from build123d import *

# Parameters (mm, degrees)
F0_W      = 80
F0_H      = 80
F1_DEPTH  = 20
F2_W      = 75
F2_H      = 75
F3_DEPTH  = 15
F4_R      = 2.5
F4_R_2    = 1.5
F5_DEPTH  = 12
F6_W      = 7.5
F6_H      = 7.5
F7_DEPTH  = 7.5
F8_R      = 2.5
F9_DEPTH  = 15
F10_SIZE2 = 1.4004150764
F10_SIZE  = 2


with BuildPart() as f1:
    # F0 (on Top) → F1 (new body)
    with BuildSketch(Plane.XY):
        Rectangle(F0_W, F0_H)
    extrude(amount=F1_DEPTH)

    # F2 (on face) → F3 (cut)
    with BuildSketch(Plane.XY.offset(20)):
        Rectangle(F2_W, F2_H)
    extrude(amount=-F3_DEPTH, mode=Mode.SUBTRACT)

    # F4 (on face) → F5 (join)
    with BuildSketch(Plane.XY.offset(5)):
        with Locations((-11, 26.5)):
            Circle(F4_R)
        with Locations((-11, 26.5)):
            Circle(F4_R_2, mode=Mode.SUBTRACT)
        with Locations((11, 26.5)):
            Circle(F4_R)
        with Locations((11, 26.5)):
            Circle(F4_R_2, mode=Mode.SUBTRACT)
        with Locations((-11, -26.5)):
            Circle(F4_R)
        with Locations((-11, -26.5)):
            Circle(F4_R_2, mode=Mode.SUBTRACT)
        with Locations((11, -26.5)):
            Circle(F4_R)
        with Locations((11, -26.5)):
            Circle(F4_R_2, mode=Mode.SUBTRACT)
        with Locations((-32.5, 18)):
            Circle(F4_R)
        with Locations((-32.5, 18)):
            Circle(F4_R_2, mode=Mode.SUBTRACT)
        with Locations((-32.5, 0)):
            Circle(F4_R)
        with Locations((-32.5, 0)):
            Circle(F4_R_2, mode=Mode.SUBTRACT)
        with Locations((-32.5, -18)):
            Circle(F4_R)
        with Locations((-32.5, -18)):
            Circle(F4_R_2, mode=Mode.SUBTRACT)
        with Locations((32.5, 0)):
            Circle(F4_R)
        with Locations((32.5, 0)):
            Circle(F4_R_2, mode=Mode.SUBTRACT)
        with Locations((32.5, -18)):
            Circle(F4_R)
        with Locations((32.5, -18)):
            Circle(F4_R_2, mode=Mode.SUBTRACT)
        with Locations((32.5, 18)):
            Circle(F4_R)
        with Locations((32.5, 18)):
            Circle(F4_R_2, mode=Mode.SUBTRACT)
    extrude(amount=F5_DEPTH)

    # F6 (on face) → F7 (join)
    with BuildSketch(Plane(origin=(-40, 0, 0), x_dir=(0, -1, 0), z_dir=(-1, 0, 0))):
        with Locations((35, 15)):
            Rectangle(F6_W, F6_H)
        with Locations((-5, 15)):
            Rectangle(F6_W, F6_H)
    extrude(amount=F7_DEPTH)

    # F8 (on face) → F9 (join)
    with BuildSketch(Plane(origin=(0, -31.25, 0), x_dir=(-1, 0, 0), z_dir=(0, 1, 0))):
        with Locations((43.75, 15)):
            Circle(F8_R)
    extrude(amount=F9_DEPTH)

    # F10
    f10_edges = [f1.edges().sort_by_distance(p)[0] for p in [
        (-41.25, -16.25, 15),
    ]]
    f10_side = f1.faces().sort_by_distance((-43.75, -16.25, 15))[0]
    chamfer(f10_edges, length=F10_SIZE, length2=F10_SIZE2, reference=f10_side)


solid = f1.part
Here's how the part is built. I have some questions about the finished solid (model axes, mm). A direction names the side the tool comes from. Coordinates: 2 decimals unless noted, no trailing zeros. Order: outer loops, then holes, each group sorted by start corner. A loop starts at its lowest first (then second) coordinate and runs counter-clockwise, first axis right, second up. Notation, with made-up numbers: (-2.75, -34.75) - (26.25, -34.75) arc R23 ccw to (26.25, -23.75) - close; hole circle Ø1 at (32.25, 62). An arc over 180 degrees is marked (long way). Use CSV: the item, a comma, the result in double quotes. Start each with the question number.
1. Suppose I cut it at A-A on y = -22.5. List the corners of the cut face in (x, z) for me, then the cut area to 3 significant figures.
2. For faces 1 (the face through (-35, -18, 11)), 2 (the face through (40, -1, 10)), 3 (the face through (-44, 5, 18.75)), 4 (the face through (-46.06, -24.55, 14.04)), which set-ups out of +Z, -Z, +X, -X, +Y, -Y let a thin tool reach every point of the face, with its end or its side?
3. Please list where these lines run through material, in increasing order: line 1 (Y direction, x = 11, z = 13.5); line 2 (Y direction, x = 22.5, z = 13.25). Write a range as from..to.
4. Suppose I cut it at B-B on x = 26.5. List the corners of the cut face in (y, z) for me.
5. I'm going to push flat-ended pins straight in: pin 1 (8 mm diameter, centred on x = -27.5, y = -28.5, fed in from +Z); pin 2 (1.5 mm diameter, centred on x = -32.5, y = 17, fed in from +Z); pin 3 (4 mm diameter, centred on y = -26.5, z = 6.5, fed in from -X); pin 4 (5 mm diameter, centred on x = -35.5, y = 7.5, fed in from +Z). Where does each tip first touch, or does it pass through?
6. If we mould it in two halves opening along Y, with no side actions, what happens to faces 5 (the face through (-1, 1, 0)), 6 (the face through (-11, 28, 11))? For each: +Y half, -Y half, draft (parallel to the pull), parting line (faces both ways), or undercut.
7. Suppose I cut it at D-D on x = 11. List the corners of the cut face in (y, z) for me, then the cut area to 3 significant figures.
Output:
1,outline,"circle Ø5 at (-43.75, 15); (-40, 0) - (40, 0) - (40, 20) - (37.5, 20) - (37.5, 5) - (-37.5, 5) - (-37.5, 20) - (-40, 20) - close"
1,area,"495 mm2"
2,face 1,"+Z"
2,face 2,"+Z, -Z, +X, +Y, -Y"
2,face 3,"+Z, -X, +Y, -Y"
2,face 4,"none"
3,line 1,"y = -40..-37.5, -29..-28, -25..-24, 24..25, 28..29, 37.5..40"
3,line 2,"y = -40..-37.5, 37.5..40"
4,outline,"(-40, 0) - (40, 0) - (40, 20) - (37.5, 20) - (37.5, 5) - (-37.5, 5) - (-37.5, 20) - (-40, 20) - close"
5,pin 1,"stops at z = 5"
5,pin 2,"stops at z = 17"
5,pin 3,"stops at x = -40"
5,pin 4,"stops at z = 20"
6,face 5,"draft"
6,face 6,"undercut"
7,outline,"(-40, 0) - (40, 0) - (40, 20) - (37.5, 20) - (37.5, 5) - (29, 5) - (29, 17) - (28, 17) - (28, 5) - (25, 5) - (25, 17) - (24, 17) - (24, 5) - (-24, 5) - (-24, 17) - (-25, 17) - (-25, 5) - (-28, 5) - (-28, 17) - (-29, 17) - (-29, 5) - (-37.5, 5) - (-37.5, 20) - (-40, 20) - close"
7,area,"523 mm2"
